Model file for the job. Use its own axes, mm. A direction names the side the tool comes from. Give positions to 0.01 mm unless a question says otherwise; leave off trailing zeros. Write each loop counter-clockwise with the first axis right and the second up, starting at its lowest first coordinate (ties: lowest second). Pieces come first, ordered by that corner, then holes. Notation, with made-up numbers: (43, 5) - (72, 5) arc R21 cw to (72, 36) - close; hole circle Ø1 at (-31.5, 10.25). An arc over 180 degrees is marked (long way). Use CSV: the item, a comma, the result in double quotes.
Autodesk Inventor part; units mm, degrees
ref_plane "YZ Plane" through (0, 0, 0) normal (1, 0, 0) x (0, 1, 0)
ref_plane "XZ Plane" through (0, 0, 0) normal (0, 1, 0) x (-1, 0, 0)
ref_plane "XY Plane" through (0, 0, 0) normal (0, 0, 1) x (1, 0, 0)
sketch "スケッチ1" plane through (0, 0, 0) normal (1, 0, 0) x (0, 1, 0)
  line L0 (12, 0) -> (12, -7)
  line L1 (22, -7) -> (22, -4)
  line L2 (22, -4) -> (20, -4)
  line L3 (20, -4) -> (20, 0)
  line L4 (20, 0) -> (12, 0)
  line L5 (0, -8.4) -> (0, 1.4)
  line L6 (22, -7) -> (12, -7)
  point P0 (0, 0)
  dimension "d0" = 20
  dimension "d1" = 2
  dimension "d2" = 4
  dimension "d3" = 3
  dimension "d4" = 8
revolve "回転1" add sketch "スケッチ1" angle 360 about axis through (0, 0, -10) along (0, 0, 1)
sketch "スケッチ2" plane through (0, 0, 0) normal (0, 0, 1) x (1, 0, 0)
  circle A0 centre (0, 0) radius 20
  circle A1 centre (0, 0) radius 16
  point P0 (0, 16)
  point P1 (-13.8564, 8)
  point P2 (-13.8564, -8)
  point P3 (0, -16)
  point P4 (13.8564, -8)
  point P5 (13.8564, 8)
  dimension "d8" = 4
  dimension "d11" = 360
hole "穴1" at (0, 16, 0) at (-13.8564, 8, 0) at (-13.8564, -8, 0) at (0, -16, 0) at (13.8564, -8, 0) at (13.8564, 8, 0) direction (0, 0, -1) diameter 3.2 end through all
chamfer "面取り1" distance 1 angle 45 1 edges at (0, -20, 0)
sketch "スケッチ3" plane through (0, 0, -7) normal (0, 0, -1) x (-1, 0, 0)
  circle A0 centre (0, 0) radius 22
  circle A1 centre (0, 0) radius 24
  line L0 (0, 0) -> (23.6354, -4.1676)
  line L1 (0, 0) -> (23.6354, 4.1676)
  line L2 (-35, 0) -> (35, 0)
  point P0 (21.6658, -3.8203)
  point P1 (21.6658, 3.8203)
  dimension "d23" = 2
  dimension "d24" = 10
  dimension "d25" = 10
extrude "押し出し1" add sketch "スケッチ3" against normal up to surface (3 mm away) contours L2 A1 L0 A0 | A0 L1 A1 L2 picked at (23.0463, -3.5914) picked at (23.1081, 3.1693)
fillet "フィレット1" radius 0.5 4 edges at (-23.6354, -4.1676, -5.5) (-21.6658, -3.8203, -5.5) (-23.6354, 4.1676, -5.5) (-21.6658, 3.8203, -5.5)
equation "\"d25\" = d24"
properties part number "base11" material "ABS プラスチック"
(1) Flat gauge pins, fed straight in: P1, Ø3, axis at x = 17, z = -5.5, coming from the -Y side; P2, Ø3, axis at x = 0, y = 16, coming from the +Z side; P3, Ø4, axis at x = -10.5, z = -5.5, coming from the +Y side; P4, Ø1.5, axis at y = 16, z = -5.5, coming from the +X side. Where does each tip first touch, or does it go through?
Checked values:
P1,"stops at y = -15.61"
P2,"passes through"
P3,"stops at y = 20.29"
P4,"stops at x = 15.86"
(2) Saw through at C-C, the plane y = 8. Count the separate pieces of the cut face and the enclosed holes in it, then the cut area to 3 significant figures.
Checked values:
separate pieces,"4"
enclosed holes,"0"
area,"98.5 mm^2"
(3) Wall check: probe 1 along Y at (x, z) = (0, -3); probe 2 along Y at (x, z) = (0, -4.5); probe 3 along Y at (x, z) = (12.5, -5.25). Give the ranges that are in metal, low to high. Write a range as [from, to].
Checked values:
probe 1,"y = [-20, -17.6], [-14.4, -12], [12, 14.4], [17.6, 20]"
probe 2,"y = [-22, -17.6], [-14.4, -12], [12, 14.4], [17.6, 22]"
probe 3,"y = [-18.1, -8.85], [-7.15, 7.15], [8.85, 18.1]"
(4) Saw through at B-B, the plane y = 0. List the corners of the cut face in (x, z).
Checked values:
outline,"(-24, -7) - (-12, -7) - (-12, 0) - (-19, 0) - (-20, -1) - (-20, -4) - (-24, -4) - close; (12, -7) - (22, -7) - (22, -4) - (20, -4) - (20, -1) - (19, 0) - (12, 0) - close"
(5) Pull direction Y, two halves, no side cores. Call faces 4 (the face through (-22.638, 3.992, -5.521)), 5 (the face through (-0.07, -14.4, -3.55)), 6 (the face through (-20, -3, -4)): released by +Y, released by -Y, zero draft, split by the parting line, or undercut.
Checked values:
face 4,"released by +Y"
face 5,"undercut"
face 6,"zero draft"
(6) Saw through at A-A, the plane x = 0. List the corners of the cut face in (y, z).
Checked values:
outline,"(-22, -7) - (-17.6, -7) - (-17.6, 0) - (-19, 0) - (-20, -1) - (-20, -4) - (-22, -4) - close; (-14.4, -7) - (-12, -7) - (-12, 0) - (-14.4, 0) - close; (12, -7) - (14.4, -7) - (14.4, 0) - (12, 0) - close; (17.6, -7) - (22, -7) - (22, -4) - (20, -4) - (20, -1) - (19, 0) - (17.6, 0) - close"
(7) 3-axis set-ups, long thin cutter, end or side, ignore diameter. For faces 1 (the face through (19.524, -4.336, -2.479)), 2 (the face through (0.53, -11.99, -3.55)), 3 (the face through (-22.638, -3.992, -5.521)): which of +Z, -Z, +X, -X, +Y, -Y reach the whole face in a straight line?
Checked values:
face 1,"+Z"
face 2,"+Z, -Z"
face 3,"+Z, -Z, -Y"
